Could you check a few things on this drawing? It's one solid part, dimensions in mm from its lowest x, y, z. A direction names the side the tool comes from. Coordinates: 2 decimals unless noted, no trailing zeros. Write each loop counter-clockwise with the first axis right and the second up, starting at its lowest first coordinate (ties: lowest second). Pieces come first, ordered by that corner, then holes. Notation, with made-up numbers: (54, -5) - (88, -5) arc R19 ccw to (88, 4) - close; hole circle Ø1 at (-21, 35). An arc over 180 degrees is marked (long way). Write each question's results on one line, items separated by ' | '. Start each with the question number.
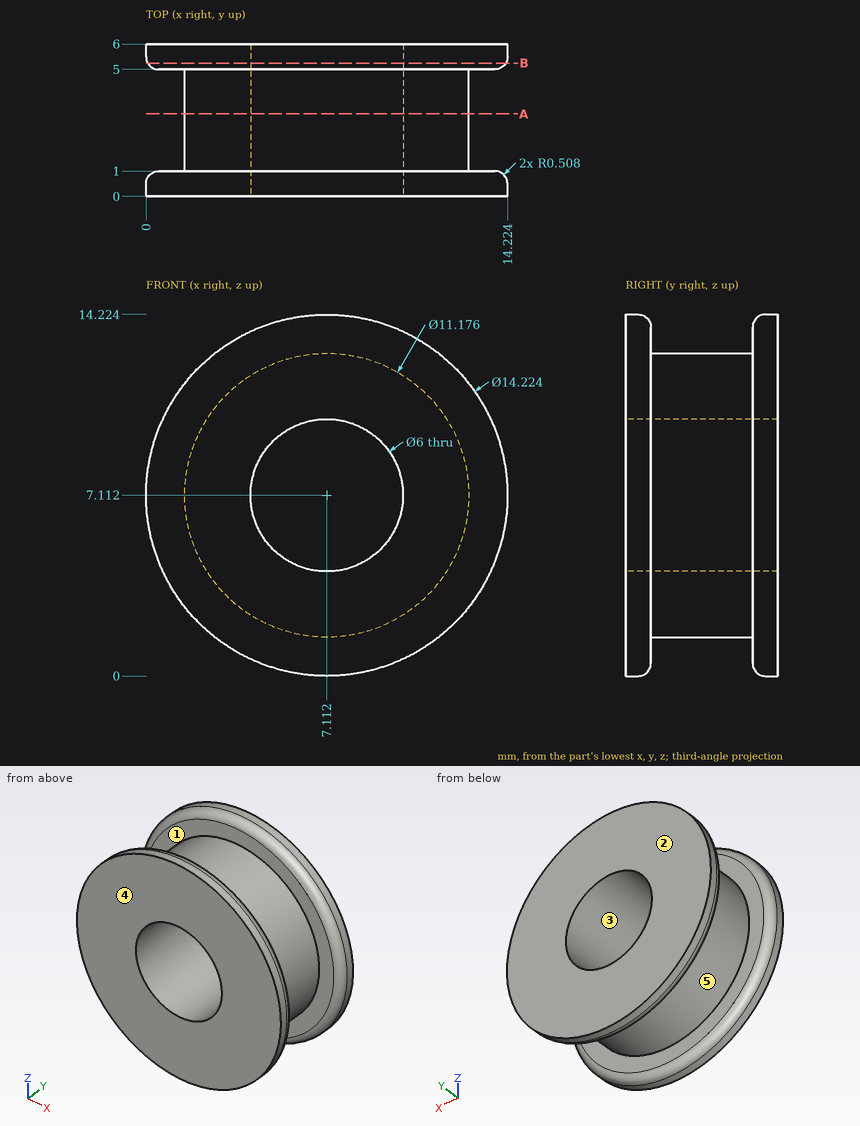
Q1. If we section it at B-B (y = 5.25): Please give me the cut outline in (x, z).
Q2. If we section it at A-A (y = 3.25): Please give me the cut outline in (x, z).
Q3. Thinking about a two-plate mould opening in X: for the marked faces 3, 4 and 5, which applies, pulls with the +X half, pulls with the -X half, needs draft (parallel to the pull), parting line crosses it, or undercut?
Q4. I need wall thicknesses on line 1 along Y through (x, z) = (9, 13.5); line 2 along Z through (x, y) = (8.5, 2); line 3 along X through (y, z) = (5.5, 6). Which ranges of each line are inside material? Lowest first, please. Write a range as from..to.
Q5. I'm going to push flat-ended pins straight in: pin 1 Ø1 at (x, z) = (7, 5) entering from +Y; pin 2 Ø1.5 at (y, z) = (1.5, 12) entering from -X. Where does each tip first touch, or does it pass through?
Q6. For the marked faces 1 and 2, which set-ups out of +Z, -Z, +X, -X, +Y, -Y let a thin tool reach every point of the face, with its end or its side?
Answer list:
1) outline: circle Ø14.08 at (7.11, 7.11); hole circle Ø6 at (7.11, 7.11)
2) outline: circle Ø11.18 at (7.11, 7.11); hole circle Ø6 at (7.11, 7.11)
3) face 3: undercut | face 4: needs draft | face 5: parting line crosses it
4) line 1: y = 0..1, 5..6 | line 2: z = 1.7..4.45, 9.77..12.52 | line 3: x = 0.09..4.33, 9.9..14.14
5) pin 1: passes through | pin 2: stops at x = 1.81
6) face 1: none | face 2: +Z, -Z, +X, -X, +Y
